from build123d import *
from build123d.topology import SkipClean

# Parameters (mm, degrees)
SKETCH1_R           = 9
SKETCH1_R_2         = 5
BOSS_EXTRUDE1_DEPTH = 2
SKETCH3_R           = 9
SKETCH2_R           = 6.5
SKETCH4_R           = 5
CUT_EXTRUDE1_DEPTH  = 5


with BuildPart() as part:
    # Sketch1 → Boss-Extrude1 (new body)
    with BuildSketch(Plane.XY):
        Circle(SKETCH1_R)
        Circle(SKETCH1_R_2, mode=Mode.SUBTRACT)
    extrude(amount=BOSS_EXTRUDE1_DEPTH)

    # Sketch3 → Loft1 section 0
    with BuildSketch(Plane(origin=(0, 0, 0), x_dir=(-1, 0, 0), z_dir=(0, 0, -1))):
        Circle(SKETCH3_R)
    # Sketch2 → Loft1 section 1
    with BuildSketch(Plane(origin=(0, 0, -3), x_dir=(-1, 0, 0), z_dir=(0, 0, -1))):
        Circle(SKETCH2_R)
    loft()

    # Sketch4 → Cut-Extrude1 (cut)
    with SkipClean():  # the faces are left unmerged after this step: merging them gives an invalid solid
        with BuildSketch(Plane(origin=(0, 0, -3), x_dir=(-1, 0, 0), z_dir=(0, 0, -1))):
            Circle(SKETCH4_R)
        extrude(amount=-CUT_EXTRUDE1_DEPTH, mode=Mode.SUBTRACT)


solid = part.part
Could you check a few things on this model? Use its own coordinates, in mm. Coordinates: 2 decimals unless noted, no trailing zeros. Order: outer loops, then holes, each group sorted by start corner. A loop starts at its lowest first (then second) coordinate and runs counter-clockwise, first axis right, second up. Notation, with made-up numbers: (30, 16) - (84, 16) arc R28 ccw to (84, 53) - close; hole circle Ø2 at (76.25, -26.5). An arc over 180 degrees is marked (long way). Answer in a Markdown table with one row per item. Add a question column.
(1) I need wall thicknesses on L1, parallel to Y at x = 0, z = -1.35 (3 decimals); L2, parallel to Y at x = 4, z = 1.1. Which ranges of each line are inside material? Lowest first, please.
(2) If we section it at C-C, the plane z = 0.9: Please give me the cut outline in (x, y), then the cut area to 3 significant figures.
(3) If we mould it in two halves opening along Y, with no side actions, what happens to faces 1 (the face through (1.08, -4.88, -0.54)), 2 (the face through (-1.172, 8.923, 0.986)), 3 (the face through (4, -4, 2))? For each: released by +Y, released by -Y, zero draft, split by the parting line, or undercut.
(4) If we section it at A-A, the plane x = 0: Please give me the cut outline in (y, z).
(5) If we section it at B-B, the plane z = -2.6: Please give me the cut outline in (x, y), then the cut area to 3 significant figures.
(6) Will these pins go through, and if not, where does the flat tip stop? pin 1 (1 mm diameter, centred on x = -3.5, y = -0.5, fed in from -Z); pin 2 (1 mm diameter, centred on y = 1.5, z = 1.5, fed in from +X); pin 3 (1.5 mm diameter, centred on x = 4, z = 1, fed in from +Y).
Results are:
| question | item | result |
|---|---|---|
| 1 | L1 | y = -7.875 to -5, 5 to 7.875 |
| 1 | L2 | y = -8.06 to -3, 3 to 8.06 |
| 2 | outline | circle Ø18 at (0, 0); hole circle Ø10 at (0, 0) |
| 2 | area | 176 mm2 |
| 3 | face 1 | undercut |
| 3 | face 2 | split by the parting line |
| 3 | face 3 | zero draft |
| 4 | outline | (-9, 0) - (-6.5, -3) - (-5, -3) - (-5, 2) - (-9, 2) - close; (5, -3) - (6.5, -3) - (9, 0) - (9, 2) - (5, 2) - close |
| 5 | outline | circle Ø13.67 at (0, 0); hole circle Ø10 at (0, 0) |
| 5 | area | 68.2 mm2 |
| 6 | pin 1 | passes through |
| 6 | pin 2 | stops at x = 8.94 |
| 6 | pin 3 | stops at y = 8.39 |
